Can you work these out from the model? Positions are in its coordinate system, mm. A direction names the side the tool comes from. Give positions to 0.01 mm unless a question says otherwise; leave off trailing zeros. Loops run counter-clockwise (first coordinate to the right, second up) from the corner with the lowest first, then second, coordinate; pieces in that order, holes last. Notation, with made-up numbers: (-20, -33) -> (-2, -33) arc R12 cw to (-2, -21) -> close; hole circle Ø3 at (-5, -33.5). An arc over 180 degrees is marked (long way). Return JSON: item names as keys, results as strings. Group by question number.
Q1. Will these pins go through, and if not, where does the flat tip stop? pin 1 (6 mm diameter, centred on x = 0, y = 105, fed in from -Z); pin 2 (8 mm diameter, centred on x = 15, y = 42.5, fed in from -Z); pin 3 (10 mm diameter, centred on x = 5, y = 46, fed in from -Z).
Q2. Thinking about a two-plate mould opening in Z: for faces 1 (the flat face through (-2.4, 105.2, -15.716)), 2 (the cylindrical face through (1.471, 116.207, -16.888)), 3 (the flat face through (0, 10, 0)), which applies, pulls with the +Z half, pulls with the -Z half, needs draft (parallel to the pull), parting line crosses it, or undercut?
Q3. I need wall thicknesses on line 1 along Y through (x, z) = (0, 18); line 2 along Y through (x, z) = (0, -16); line 3 along Z through (x, y) = (0, 3). Which ranges of each line are inside material? Lowest first, please. Write a range as [from, to].
Q4. Suppose I cut it at B-B, the plane x = -17.5. Please give me the cut outline in (y, z).
Q5. Suppose I cut it at C-C, the plane y = 40. Please give me the cut outline in (x, z), and give its area (3 significant figures).
Q6. Suppose I cut it at A-A, the plane z = 0. Please give me the cut outline in (x, y).
Q7. Suppose I cut it at D-D, the plane z = -24.5. Please give me the cut outline in (x, y).
Q8. Which directions (+Z, -Z, +X, -X, +Y, -Y) give clear straight access to the entire face, cutting with the end or side of a thin tool? Please do faces 4 (the flat face through (0, 5, -2.111)), 5 (the flat face through (26, 106, -40.327)), 6 (the flat face through (-2.111, 105, 1)), 7 (the flat face through (21.15, 105, -29)).
Autodesk Inventor part; units mm, degrees
ref_plane "YZ Plane" through (0, 0, 0) normal (1, 0, 0) x (0, 1, 0)
ref_plane "XZ Plane" through (0, 0, 0) normal (0, 1, 0) x (-1, 0, 0)
ref_plane "XY Plane" through (0, 0, 0) normal (0, 0, 1) x (1, 0, 0)
sketch "Sketch1" plane through (0, 0, 0) normal (0, 1, 0) x (-1, 0, 0)
  circle A0 centre (0, 0) radius 40
  dimension "d0" = 80
extrude "Extrusion1" add sketch "Sketch1" along normal blind 100
sketch "Sketch2" plane through (0, 100, 0) normal (0, 1, 0) x (1, 0, 0)
  line L0 (-10.8438, 4.9816) -> (0, 4.9816)
  line L1 (0, 4.9816) -> (0, -2.1726)
  line L2 (0, -2.1726) -> (-10.8438, -2.1726)
  line L3 (-10.8438, -2.1726) -> (-10.8438, 4.9816)
  point P0 (0, 0)
extrude "Extrusion2" add sketch "Sketch2" along normal blind 10
sketch "Sketch3" plane through (-10.8438, 100, 2.1726) normal (0, 0, 1) x (1, 0, 0)
  line L0 (10.8438, 0) -> (10.8438, 10)
  circle A0 centre (10.8438, 5) radius 40
  point P0 (10.8438, -100)
  dimension "d5" = 80
extrude "Extrusion3" add sketch "Sketch3" along normal blind 38 and the other way blind 42.5
sketch "Sketch4" plane through (-10.8438, 100, 40.1726) normal (0, 0, 1) x (1, 0, 0)
  circle A0 centre (10.8438, 5) radius 2.5527
  line L0 (9.4087, 7.1111) -> (12.2789, 7.1111)
  circle A1 centre (10.8438, 5) radius 40
  point P0 (10.8438, -100)
  dimension "d10" = 5.1054
  dimension "d11" = 2.8702
extrude "Extrusion4" cut sketch "Sketch4" against normal blind 22.5044 contours A0 L0 picked at (10.9442, 5.5624)
sketch "Sketch5" plane through (0, 0, 0) normal (0, -1, 0) x (1, 0, 0)
  circle A0 centre (0, 0) radius 2.5527
  line L0 (1.4351, -2.1111) -> (-1.4351, -2.1111)
  dimension "d14" = 5.1054
  dimension "d15" = 2.8702
extrude "Extrusion5" cut sketch "Sketch5" against normal blind 10 contours A0 L0 picked at (0.1004, -0.5624)
sketch "Sketch6" plane through (0, 105, -40.3274) normal (0, 0, -1) x (-1, 0, 0)
  line L0 (-21.15, -21.15) -> (21.15, -21.15)
  line L1 (21.15, -21.15) -> (21.15, 21.15)
  line L2 (21.15, 21.15) -> (-21.15, 21.15)
  line L3 (-21.15, 21.15) -> (-21.15, -21.15)
  line L4 (-21.15, -21.15) -> (21.15, 21.15) construction
  line L5 (21.15, -21.15) -> (-21.15, 21.15) construction
  circle A0 centre (0, 0) radius 40
  point P0 (0, -105)
  dimension "d18" = 42.3
  dimension "d19" = 42.3
  dimension "d27" = 21.15
  dimension "d28" = 21.15
extrude "Extrusion6" cut sketch "Sketch6" against normal blind 22.3 contours L3 L2 L1 L0
sketch "Sketch7" plane through (0, 105, -18.0274) normal (0, 0, -1) x (-1, 0, 0)
  circle A0 centre (0, 0) radius 11.303
  circle A1 centre (0, 0) radius 40
  point P0 (0, -105)
  dimension "d22" = 22.606
extrude "Extrusion7" cut sketch "Sketch7" against normal blind 2.3114 contours A0
sketch "Sketch8" plane through (0, 105, -15.716) normal (0, 0, -1) x (-1, 0, 0)
  circle A0 centre (0, 0) radius 2.5527
  line L0 (2.1111, 1.4351) -> (2.1111, -1.4351)
  circle A1 centre (0, 0) radius 40
  point P0 (0, -105)
  dimension "d25" = 5.1054
  dimension "d26" = 2.8702
extrude "Extrusion8" cut sketch "Sketch8" against normal blind 60 contours L0 A0 picked at (0.5627, -0.1029)
Ans:
{
 "1": {"pin 1": "stops at z = -15.72", "pin 2": "stops at z = -38.46", "pin 3": "stops at z = -40"},
 "2": {"face 1": "pulls with the -Z half", "face 2": "needs draft", "face 3": "undercut"},
 "3": {"line 1": "y = [0, 102.45], [107.55, 145]", "line 2": "y = [0, 93.7], [116.3, 145]", "line 3": "z = [-40, -2.11], [2.55, 40]"},
 "4": {"outline": "(0, -35.97) -> (69.03, -35.97) -> (69.03, -40.33) -> (83.85, -40.33) -> (83.85, -18.03) -> (126.15, -18.03) -> (126.15, -40.33) -> (140.97, -40.33) -> (140.97, 40.17) -> (69.03, 40.17) -> (69.03, 35.97) -> (0, 35.97) -> close"},
 "5": {"outline": "circle Ø80 at (0, 0)", "area": "5,030 mm^2"},
 "6": {"outline": "(-40, 0) -> (-2.55, 0) -> (-2.55, 10) -> (2.55, 10) -> (2.55, 0) -> (40, 0) -> (40, 100) -> (39.69, 100) arc R40 ccw (long way) to (-39.69, 100) -> (-40, 100) -> close; hole (-2.11, 103.56) arc R2.55 ccw (long way) to (-2.11, 106.44) -> close"},
 "7": {"outline": "(-31.62, 0) -> (31.62, 0) -> (31.62, 80.5) arc R40 ccw (long way) to (-31.62, 80.5) -> close; hole (-21.15, 83.85) -> (21.15, 83.85) -> (21.15, 126.15) -> (-21.15, 126.15) -> close"},
 "8": {"face 4": "-Y", "face 5": "-Z, +X, -X, +Y, -Y", "face 6": "+Z, -Z", "face 7": "-Z"}
}
